Verification items for the finished model (mm, model axes). A direction names the side the tool comes from. Give positions to 0.01 mm unless a question says otherwise; leave off trailing zeros. Loops run counter-clockwise (first coordinate to the right, second up) from the corner with the lowest first, then second, coordinate; pieces in that order, holes last. Notation, with made-up numbers: (-19.5, 21.25) -> (17.5, 21.25) arc R22 ccw to (17.5, 35.25) -> close; hole circle Ø5 at (76, -8.75). An arc over 180 degrees is marked (long way). Answer in a Markdown table with one row per item. Add a question column.
Q1. Set-up check for faces 5 (the face through (-1.367, 1.661, -1.726)), 6 (the face through (0.07, 2.1, 10.35)), 7 (the face through (0, -0.35, 14)): record each of +Z, -Z, +X, -X, +Y, -Y from which the full face is reachable in a straight line by a thin tool's end or side.
Q2. Section check B-B on y = 0. Enter the section's corners in (x, z), and give its area (3 significant figures).
Q3. Section check C-C on z = 11.5. Enter the section's corners in (x, y).
Q4. Gauge pin test, flat ends, axial feed: P1, Ø3, axis at y = 1, z = 1.5, coming from the +X side; P2, Ø1.3, axis at x = -0.5, z = 13.5, coming from the -Y side; P3, Ø2, axis at x = -3.5, y = 1, coming from the +Z side; P4, Ø4, axis at y = -3, z = 6.5, coming from the +X side. Record the tip position at first contact, or that the pin passes through.
Q5. Material ranges on probe 1 along Z at (x, y) = (0.25, 3); probe 2 along Y at (x, z) = (-1.5, 2.75); probe 3 along X at (y, z) = (2, -1.75), recorded low to high.
Q6. Section check A-A on x = 0. Enter the section's corners in (y, z).
Q7. Release check for a two-part mould opening along X. For faces 1 (the face through (0, 0, 0)), 2 (the face through (1.346, 1.776, -1.726)), 3 (the face through (0, 0.35, 14)), 4 (the face through (-3.65, -2.8, 3.21)) record: pulls with the +X half, pulls with the -X half, needs draft (parallel to the pull), parting line crosses it, or undercut.
```python
from build123d import *

# Parameters (mm, degrees)
SKETCH_R        = 4.6
PAD_DEPTH       = 6.5
SKETCH001_R     = 0.45
PAD001_DEPTH    = 3.5
SKETCH002_R     = 2.1
PAD002_DEPTH    = 7.8
POCKET_DEPTH    = 1.2
SKETCH004_W     = 4.141256
SKETCH004_H     = 0.6
POCKET001_DEPTH = 7.8
FILLET_R        = 0.25


with BuildPart() as part:
    # Sketch → Pad (new body)
    with BuildSketch(Plane.XY):
        Circle(SKETCH_R)
    extrude(amount=PAD_DEPTH)

    # Sketch001 (on Face2 of Pad) → Pad001 (join)
    with BuildSketch(Plane(origin=(0, 0, 0), x_dir=(1, 0, 0), z_dir=(0, 0, -1))):
        with Locations((2.54, 0)):
            Circle(SKETCH001_R)
        with Locations((1.796051, 1.796051)):
            Circle(SKETCH001_R)
        with Locations((0, 2.54)):
            Circle(SKETCH001_R)
        with Locations((-1.796051, 1.796051)):
            Circle(SKETCH001_R)
        with Locations((-2.54, 0)):
            Circle(SKETCH001_R)
        with Locations((-1.796051, -1.796051)):
            Circle(SKETCH001_R)
        with Locations((0, -2.54)):
            Circle(SKETCH001_R)
        with Locations((1.796051, -1.796051)):
            Circle(SKETCH001_R)
    extrude(amount=PAD001_DEPTH)

    # Sketch002 (on Face3 of Pad001) → Pad002 (join)
    with BuildSketch(Plane.XY.offset(6.5)):
        Circle(SKETCH002_R)
    extrude(amount=PAD002_DEPTH)

    # Sketch003 (on Face21 of Pad002) → Pocket (cut)
    with BuildSketch(Plane.XY.offset(14.3)):
        with BuildLine():
            Line((-2.070628, -0.35), (2.070628, -0.35))
            ThreePointArc((2.070628, -0.35), (2.1, 0), (2.070628, 0.35))
            Line((2.070628, 0.35), (-2.070628, 0.35))
            ThreePointArc((-2.070628, 0.35), (-2.1, 0), (-2.070628, -0.35))
        make_face()
    extrude(amount=-POCKET_DEPTH, mode=Mode.SUBTRACT)

    # Sketch004 (on Face23 of Pocket) → Pocket001 (cut)
    with BuildSketch(Plane.XY.offset(14.3)):
        with Locations((0, -1.8)):
            Rectangle(SKETCH004_W, SKETCH004_H)
    extrude(amount=-POCKET001_DEPTH, mode=Mode.SUBTRACT)

    # Fillet
    fillet_edges = [part.edges().sort_by_distance(p)[0] for p in [
        (-4.6, 0, 6.5),
        (-4.6, 0, 0),
    ]]
    fillet(fillet_edges, radius=FILLET_R)


solid = part.part
```
Taken from the geometry:
| question | item | result |
|---|---|---|
| 1 | face 5 | -Z |
| 1 | face 6 | +Z |
| 1 | face 7 | +Z, +X, -X |
| 2 | outline | (-4.6, 0.25) arc R0.25 ccw to (-4.35, 0) -> (-2.99, 0) -> (-2.99, -3.5) -> (-2.09, -3.5) -> (-2.09, 0) -> (2.09, 0) -> (2.09, -3.5) -> (2.99, -3.5) -> (2.99, 0) -> (4.35, 0) arc R0.25 ccw to (4.6, 0.25) -> (4.6, 6.25) arc R0.25 ccw to (4.35, 6.5) -> (2.1, 6.5) -> (2.1, 13.1) -> (-2.1, 13.1) -> (-2.1, 6.5) -> (-4.35, 6.5) arc R0.25 ccw to (-4.6, 6.25) -> close |
| 2 | area | 93.8 mm² |
| 3 | outline | (-1.47, -1.5) -> (1.47, -1.5) arc R2.1 ccw (long way) to start |
| 4 | P1 | stops at x = 4.6 |
| 4 | P2 | stops at y = -1.5 |
| 4 | P3 | stops at z = 6.5 |
| 4 | P4 | stops at x = 4.49 |
| 5 | probe 1 | z = 0 to 6.5 |
| 5 | probe 2 | y = -4.35 to 4.35 |
| 5 | probe 3 | x = -2.2 to -1.39, 1.39 to 2.2 |
| 6 | outline | (-4.6, 0.25) arc R0.25 ccw to (-4.35, 0) -> (-2.99, 0) -> (-2.99, -3.5) -> (-2.09, -3.5) -> (-2.09, 0) -> (2.09, 0) -> (2.09, -3.5) -> (2.99, -3.5) -> (2.99, 0) -> (4.35, 0) arc R0.25 ccw to (4.6, 0.25) -> (4.6, 6.25) arc R0.25 ccw to (4.35, 6.5) -> (2.1, 6.5) -> (2.1, 14.3) -> (0.35, 14.3) -> (0.35, 13.1) -> (-0.35, 13.1) -> (-0.35, 14.3) -> (-1.5, 14.3) -> (-1.5, 6.5) -> (-4.35, 6.5) arc R0.25 ccw to (-4.6, 6.25) -> close |
| 7 | face 1 | undercut |
| 7 | face 2 | undercut |
| 7 | face 3 | needs draft |
| 7 | face 4 | parting line crosses it |
